Geometry: final body of the model. Coordinates: model frame, mm. A direction names the side the tool comes from. Round coordinates to 2 decimals unless told otherwise and drop trailing zeros. Write each loop counter-clockwise with the first axis right and the second up, starting at its lowest first coordinate (ties: lowest second). Pieces come first, ordered by that corner, then holes.
from build123d import *

# Parameters (mm, degrees)
F1_W     = 45
F1_H     = 35
F1_R     = 1.75
F2_DEPTH = 3.5
F3_R     = 1.75
F4_DEPTH = 1.5


with BuildPart() as f2:
    # F1 (on face) → F2 (new body)
    with BuildSketch(Plane.XY):
        with Locations((-32.283769, -12.20101)):
            Rectangle(F1_W, F1_H)
        with Locations((-49.70004, -24.70101)):
            Circle(F1_R, mode=Mode.SUBTRACT)
        with Locations((-14.867499, -24.70101)):
            Circle(F1_R, mode=Mode.SUBTRACT)
        with Locations((-49.70004, 0.29899)):
            Circle(F1_R, mode=Mode.SUBTRACT)
        with Locations((-14.867499, 0.29899)):
            Circle(F1_R, mode=Mode.SUBTRACT)
    extrude(amount=F2_DEPTH)

    # F3 (on face) → F4 (cut)
    with BuildSketch(Plane.XY.offset(3.5)):
        Polygon((-45.658588, -24.70101), (-47.679314, -21.20101), (-51.720766, -21.20101), (-53.741492, -24.70101), (-51.720766, -28.20101), (-47.679314, -28.20101), align=None)
        with Locations((-49.70004, -24.70101)):
            Circle(F3_R, mode=Mode.SUBTRACT)
        Polygon((-45.658588, 0.29899), (-47.679314, 3.79899), (-51.720766, 3.79899), (-53.741492, 0.29899), (-51.720766, -3.20101), (-47.679314, -3.20101), align=None)
        with Locations((-49.70004, 0.29899)):
            Circle(F3_R, mode=Mode.SUBTRACT)
        Polygon((-16.888224, 3.79899), (-18.90895, 0.29899), (-16.888224, -3.20101), (-12.846773, -3.20101), (-10.826047, 0.29899), (-12.846773, 3.79899), align=None)
        with Locations((-14.867499, 0.29899)):
            Circle(F3_R, mode=Mode.SUBTRACT)
        Polygon((-12.846773, -21.20101), (-16.888224, -21.20101), (-18.90895, -24.70101), (-16.888224, -28.20101), (-12.846773, -28.20101), (-10.826047, -24.70101), align=None)
        with Locations((-14.867499, -24.70101)):
            Circle(F3_R, mode=Mode.SUBTRACT)
    extrude(amount=-F4_DEPTH, mode=Mode.SUBTRACT)


solid = f2.part
1) Reachability of faces 1 (the flat face through (-17.91, -26.43, 2.76)), 2 (the cylindrical face through (-13.198, 0.825, 0.986)) from +Z, -Z, +X, -X, +Y, -Y: full face, straight path, thin tool, end or side. Return the list, or none.
2) Draft query along Y for faces 3 (the flat face through (-33, -12, 3.5)), 4 (the flat face through (-47.96, -23.87, 2)). Return one class per face: pulls with the +Y half, pulls with the -Y half, needs draft (parallel to the pull), parting line crosses it, or undercut.
3) Line query: probe 1 along Y at (x, z) = (-14, 0.95); probe 2 along Y at (x, z) = (-15, 3.3); probe 3 along X at (y, z) = (-23, 2.05). Output: solid intervals per line, ascending.
4) Section B-B on y = 1. Output: boundary loops of the cut face in (x, z).
5) Section A-A on z = 1. Output: boundary loops of the cut face in (x, y), plus the area to 3 significant figures.
6) First-contact query: P1, Ø2, axis at x = -51, y = 1.5, coming from the +Z side. Flat tip, straight axial feed; report the tip coordinate or a pass-through.
Filled in:
1. face 1: +Z
1. face 2: +Z, -Z
2. face 3: needs draft
2. face 4: undercut
3. probe 1: y = -29.7 to -26.22, -23.18 to -1.22, 1.82 to 5.3
3. probe 2: y = -29.7 to -28.2, -21.2 to -3.2, 3.8 to 5.3
3. probe 3: x = -54.78 to -52.76, -46.64 to -17.93, -11.81 to -9.78
4. outline: (-54.78, 0) - (-51.3, 0) - (-51.3, 2) - (-53.34, 2) - (-53.34, 3.5) - (-54.78, 3.5) - close; (-48.1, 0) - (-16.47, 0) - (-16.47, 2) - (-18.5, 2) - (-18.5, 3.5) - (-46.06, 3.5) - (-46.06, 2) - (-48.1, 2) - close; (-13.26, 0) - (-9.78, 0) - (-9.78, 3.5) - (-11.23, 3.5) - (-11.23, 2) - (-13.26, 2) - close
5. outline: (-54.78, -29.7) - (-9.78, -29.7) - (-9.78, 5.3) - (-54.78, 5.3) - close; hole circle Ø3.5 at (-49.7, -24.7); hole circle Ø3.5 at (-49.7, 0.3); hole circle Ø3.5 at (-14.87, -24.7); hole circle Ø3.5 at (-14.87, 0.3)
5. area: 1,540 mm2
6. P1: stops at z = 2
